Can you work these out from the model? Positions are in its coordinate system, mm. Coordinates: 2 decimals unless noted, no trailing zeros. Write each loop counter-clockwise with the first axis right and the second up, starting at its lowest first coordinate (ties: lowest second). Pieces come first, ordered by that corner, then holes. Notation, with made-up numbers: (-17, -10) -> (22, -10) arc R20 ccw to (22, 28) -> close; hole circle Ø10 at (46.25, 5.5). An arc over 180 degrees is marked (long way). Use one line per item in the form item = value.
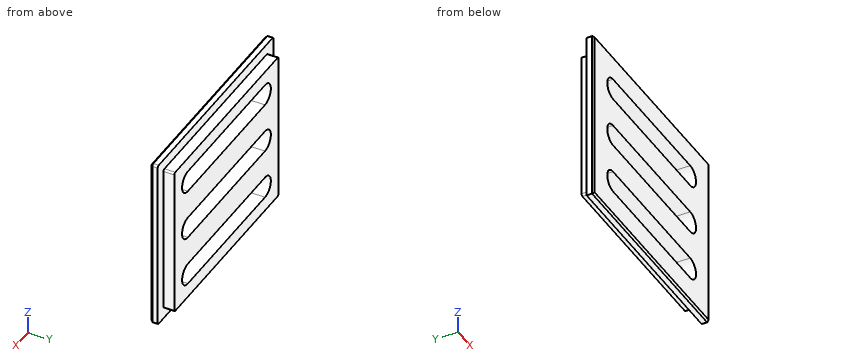
```python
from build123d import *

# Parameters (mm, degrees)
SKETCH1_W           = 60
SKETCH1_H           = 48
BOSS_EXTRUDE1_DEPTH = 2
SKETCH2_W           = 54
SKETCH2_H           = 42
BOSS_EXTRUDE2_DEPTH = 3
CUT_EXTRUDE1_DEPTH  = 50
FILLET1_R           = 0.5
CHAMFER1_SIZE       = 0.5


with BuildPart() as part:
    # Sketch1 → Boss-Extrude1 (new body)
    with BuildSketch(Plane(origin=(0, 0, 0), x_dir=(1, 0, 0), z_dir=(0, 1, 0))):
        Rectangle(SKETCH1_W, SKETCH1_H)
    extrude(amount=BOSS_EXTRUDE1_DEPTH)

    # Sketch2 → Boss-Extrude2 (add)
    with BuildSketch(Plane(origin=(0, 2, 0), x_dir=(1, 0, 0), z_dir=(0, 1, 0))):
        Rectangle(SKETCH2_W, SKETCH2_H)
    extrude(amount=BOSS_EXTRUDE2_DEPTH)

    # Sketch4 → Cut-Extrude1 (cut)
    with BuildSketch(Plane(origin=(0, 5, 0), x_dir=(1, 0, 0), z_dir=(0, 1, 0))):
        with BuildLine():
            Line((-20, -3), (20, -3))
            ThreePointArc((20, -3), (23, 0), (20, 3))
            Line((20, 3), (-20, 3))
            ThreePointArc((-20, 3), (-23, 0), (-20, -3))
        make_face()
        with BuildLine():
            Line((-20, 11), (20, 11))
            ThreePointArc((20, 11), (23, 14), (20, 17))
            Line((20, 17), (-20, 17))
            ThreePointArc((-20, 17), (-23, 14), (-20, 11))
        make_face()
        with BuildLine():
            Line((-20, -17), (20, -17))
            ThreePointArc((20, -17), (23, -14), (20, -11))
            Line((20, -11), (-20, -11))
            ThreePointArc((-20, -11), (-23, -14), (-20, -17))
        make_face()
    extrude(amount=-CUT_EXTRUDE1_DEPTH, mode=Mode.SUBTRACT)

    # Fillet1
    fillet1_edges = [part.edges().sort_by_distance(p)[0] for p in [
        (-27, 3.5, -21),
        (-27, 3.5, 21),
        (27, 3.5, 21),
        (27, 3.5, -21),
        (30, 1, -24),
        (30, 1, 24),
        (-30, 1, 24),
    ]]
    fillet(fillet1_edges, radius=FILLET1_R)

    # Chamfer1
    chamfer1_edges = [part.edges().sort_by_distance(p)[0] for p in [
        (-30, 0, -0.25),
        (0, 0, 24),
        (-0.25, 0, -24),
        (30, 0, 0),
        (29.853553391, 0, -23.853553391),
        (29.853553391, 0, 23.853553391),
        (-29.853553391, 0, 23.853553391),
    ]]
    chamfer(chamfer1_edges, length=CHAMFER1_SIZE - 0.0001)  # a hair under: the kernel refuses the full size


solid = part.part
```
Q1. Suppose I cut it at C-C (y = 3.4). Write out the boundary of the cut face in (x, z), then the cut area to 3 significant figures.
Return value:
outline = (-27, -20.5) arc R0.5 ccw to (-26.5, -21) -> (26.5, -21) arc R0.5 ccw to (27, -20.5) -> (27, 20.5) arc R0.5 ccw to (26.5, 21) -> (-26.5, 21) arc R0.5 ccw to (-27, 20.5) -> close; hole (-20, -17) -> (20, -17) arc R3 ccw to (20, -11) -> (-20, -11) arc R3 ccw to start; hole (-20, -3) -> (20, -3) arc R3 ccw to (20, 3) -> (-20, 3) arc R3 ccw to start; hole (-20, 11) -> (20, 11) arc R3 ccw to (20, 17) -> (-20, 17) arc R3 ccw to start
area = 1,460 mm2
Q2. Suppose I cut it at A-A (z = -14). Write out the boundary of the cut face in (x, y), then the cut area to 4 significant figures.
Return value:
outline = (-30, 0.5) -> (-29.5, 0) -> (-23, 0) -> (-23, 5) -> (-27, 5) -> (-27, 2) -> (-30, 2) -> close; (23, 0) -> (29.5, 0) -> (30, 0.5) -> (30, 2) -> (27, 2) -> (27, 5) -> (23, 5) -> close
area = 51.75 mm2
Q3. Suppose I cut it at B-B (x = 8). Write out the boundary of the cut face in (y, z).
Return value:
outline = (0, -23.5) -> (0.5, -24) -> (2, -24) -> (2, -21) -> (5, -21) -> (5, -17) -> (0, -17) -> close; (0, -11) -> (5, -11) -> (5, -3) -> (0, -3) -> close; (0, 3) -> (5, 3) -> (5, 11) -> (0, 11) -> close; (0, 17) -> (5, 17) -> (5, 21) -> (2, 21) -> (2, 24) -> (0.5, 24) -> (0, 23.5) -> close
Q4. Will these pins go through, and if not, where does the flat tip stop? pin 1 (2.5 mm diameter, centred on y = 4, z = 0.5, fed in from +X); pin 2 (0.9 mm diameter, centred on x = -2.5, y = 3.5, fed in from -Z); pin 3 (0.9 mm diameter, centred on x = 6, y = 3, fed in from +Z).
Return value:
pin_1 = 27
pin_2 = -21
pin_3 = 21
Q5. Suppose I cut it at D-D (z = 8). Write out the boundary of the cut face in (x, y).
Return value:
outline = (-30, 0.5) -> (-29.5, 0) -> (29.5, 0) -> (30, 0.5) -> (30, 2) -> (27, 2) -> (27, 5) -> (-27, 5) -> (-27, 2) -> (-30, 2) -> close
Q6. If I drill on line 1 (Z direction, x = 1.5, y = 0.7); line 2 (Z direction, x = -8.5, y = 3.7); line 3 (X direction, y = 2.9, z = 14), over which ranges is the centre line in solid material (lowest first)? Write a range as from..to.
Return value:
line_1 = -24..-17, -11..-3, 3..11, 17..24
line_2 = -21..-17, -11..-3, 3..11, 17..21
line_3 = -27..-23, 23..27
